```python
from build123d import *

# Parameters (mm, degrees)
F1_DEPTH = 63.5
F2_DEPTH = 25.4
F3_DEPTH = 7.9375
F5_R     = 5.08


with BuildPart() as f1:
    # F0 (on Front) → F1 (new body, symmetric)
    with BuildSketch(Plane.XZ):
        Polygon((22.225, 9.525), (-41.275, 9.525), (-41.275, -9.525), (41.275, -9.525), (41.275, 9.525), align=None)
    extrude(amount=F1_DEPTH, both=True)

    # F0 (on Front) → F2 (join, symmetric)
    with BuildSketch(Plane.XZ):
        Polygon((83.458367, 61.9252), (60.325, 61.9252), (60.325, 42.8752), (83.458367, 42.8752), (85.725, 42.8752), (85.725, 61.9252), align=None)
        with BuildLine():
            Line((22.225, 27.055343), (22.225, 9.525))
            Line((22.225, 9.525), (41.275, 9.525))
            Line((41.275, 9.525), (41.275, 27.055343))
            ThreePointArc((41.275, 27.055343), (46.402245, 38.738724), (58.472026, 42.8752))
            Line((58.472026, 42.8752), (60.325, 42.8752))
            Line((60.325, 42.8752), (60.325, 61.9252))
            Line((60.325, 61.9252), (59.111812, 61.9252))
            add(Edge.make_bspline(
                [(53.39808, 61.778228), (55.302948, 61.866382), (57.208525, 61.91594), (59.111812, 61.9252)],
                knots=[108.876649, 108.876649, 108.876649, 108.876649, 113.239979, 113.239979, 113.239979, 113.239979], degree=3))
            ThreePointArc((53.39808, 61.778228), (31.161623, 50.386865), (22.225, 27.055343))
        make_face()
    extrude(amount=F2_DEPTH, both=True)

    # F0 (on Front) → F3 (join, symmetric)
    with BuildSketch(Plane.XZ):
        with BuildLine():
            add(Edge.make_bspline(
                [(-41.275, 9.525), (-41.223468, 33.347389), (5.866576, 59.578541), (53.39808, 61.778228)],
                knots=[0, 0, 0, 0, 108.876649, 108.876649, 108.876649, 108.876649], degree=3))
            Line((-41.275, 9.525), (22.225, 9.525))
            Line((22.225, 9.525), (22.225, 27.055343))
            ThreePointArc((22.225, 27.055343), (31.161623, 50.386865), (53.39808, 61.778228))
        make_face()
    extrude(amount=F3_DEPTH, both=True)

    # F0 (on Front) → F4 (revolve)
    with BuildSketch(Plane.XZ):
        Polygon((111.125, 66.675), (85.725, 66.675), (85.725, 61.9252), (85.725, 42.8752), (85.725, 38.1), (111.125, 38.1), align=None)
    revolve(axis=Axis((85.725, 0, 52.3875), (0, 0, -1)))

    # F5
    f5_edges = [f1.edges().sort_by_distance(p)[0] for p in [
        (41.275, -63.5, 0),
        (-41.275, -63.5, 0),
        (-41.275, 63.5, 0),
        (41.275, 63.5, 0),
    ]]
    fillet(f5_edges, radius=F5_R)


solid = f1.part
```
For this review, take the finished solid that the model builds, in its own axes (mm). A direction names the side the tool comes from. Coordinates: 2 decimals unless noted, no trailing zeros. Loops run counter-clockwise (first coordinate to the right, second up) from the corner with the lowest first, then second, coordinate; pieces in that order, holes last. Notation, with made-up numbers: (-10.75, -39.75) -> (7.25, -39.75) arc R16 ccw to (7.25, -31.75) -> close; hole circle Ø3 at (47.25, -24). An arc over 180 degrees is marked (long way). Return JSON: item names as keys, results as strings. Group by question number.
(1) Tool access review of faces 5 (the flat face through (60, -2, 42.875)), 6 (the flat face through (46, 25.4, 42)), 7 (the flat face through (-4, 7.938, 30)): name each direction out of +Z, -Z, +X, -X, +Y, -Y from which nothing blocks a thin tool from reaching the whole face with its end or side.
(2) For pin 1 Ø4 at (y, z) = (-16, 48.5) entering from +X; pin 2 Ø1 at (y, z) = (-22.5, 34) entering from +X; pin 3 Ø8.5 at (y, z) = (-19.5, 15) entering from -X (3 decimals), all flat-tipped, find the tip position at first contact; note any pin that passes through.
(3) To check wall thickness, follow L1, parallel to Z at x = 18.5, y = -17.5 (3 decimals); L2, parallel to Z at x = 66, y = 22.5; L3, parallel to X at y = -20, z = 28. State the ranges of each line that lie inside material, in increasing order.
(4) Mouldability with a two-part tool opening along X and no side actions: class faces 1 (the cylindrical face through (31.4, -16.79, 50.65)), 2 (the cylindrical face through (39.8, 62, 0.1)), 3 (the flat face through (1, 35, 9.525)), 4 (the cylindrical face through (46.268, -0.356, 38.613)) as pulls with the +X half, pulls with the -X half, needs draft (parallel to the pull), parting line crosses it, or undercut.
(5) Consider section C-C, the plane x = 95. Give the boundary of the cut face in (y, z) (3 decimals), plus the area to 3 significant figures.
(6) Consider section B-B, the plane y = -41.5. Give the boundary of the cut face in (x, z) (3 decimals), plus the area to 3 significant figures.
(7) Consider section A-A, the plane x = 63. Give the boundary of the cut face in (y, z) (3 decimals).
Results below:
{
 "1": {"face 5": "-Z", "face 6": "+Z, +X, -X, +Y", "face 7": "+Z, -X, +Y"},
 "2": {"pin 1": "stops at x = 106.92", "pin 2": "stops at x = 43.13", "pin 3": "stops at x = 22.225"},
 "3": {"L1": "z = -9.525 to 9.525", "L2": "z = 42.88 to 61.93", "L3": "x = 22.24 to 41.3"},
 "4": {"face 1": "pulls with the -X half", "face 2": "pulls with the +X half", "face 3": "needs draft", "face 4": "undercut"},
 "5": {"outline": "(-23.646, 38.1) -> (23.646, 38.1) -> (23.646, 66.675) -> (-23.646, 66.675) -> close", "area": "1,350 mm2"},
 "6": {"outline": "(-41.275, -9.525) -> (41.275, -9.525) -> (41.275, 9.525) -> (-41.275, 9.525) -> close", "area": "1,570 mm2"},
 "7": {"outline": "(-25.4, 42.875) -> (-11.346, 42.875) -> (-11.346, 38.1) -> (11.346, 38.1) -> (11.346, 42.875) -> (25.4, 42.875) -> (25.4, 61.925) -> (11.346, 61.925) -> (11.346, 66.675) -> (-11.346, 66.675) -> (-11.346, 61.925) -> (-25.4, 61.925) -> close"}
}
